Check sheet for the drawn part. Datum: minimum x, y, z corner. Units: mm. A direction names the side the tool comes from. Give positions to 0.01 mm unless a question says otherwise; leave off trailing zeros. Loops run counter-clockwise (first coordinate to the right, second up) from the corner with the lowest first, then second, coordinate; pieces in that order, holes last.
1. Cross-section at C-C, the plane x = 22. Record the cut outline in (y, z).
2. Cross-section at D-D, the plane z = 17. Record the cut outline in (x, y), plus the area to 3 significant figures.
3. Cross-section at A-A, the plane z = 6.5. Record the cut outline in (x, y).
4. Cross-section at B-B, the plane x = 5.5. Record the cut outline in (y, z).
5. Material ranges on L1, parallel to Z at x = 38.5, y = 16.75; L2, parallel to X at y = 11, z = 32; L3, parallel to X at y = 15.75, z = 32, recorded low to high.
6. Go/stop test with flat-tipped pins: pin 1 Ø4.5 at (x, z) = (5.5, 32.5) entering from +Y; pin 2 Ø10.5 at (x, z) = (38, 21) entering from -Y; pin 3 Ø14 at (x, y) = (22, 15) entering from -Z; pin 4 Ø1.5 at (x, z) = (12.5, 8) entering from -Y. Record where each tip stops, or that it passes through.
7. Release check for a two-part mould opening along Y. For the marked faces 4, 5 and 6 record: +Y half, -Y half, draft (parallel to the pull), parting line (faces both ways), or undercut.
8. Tool access check on the marked faces 1, 2 and 3. Record the directions out of +Z, -Z, +X, -X, +Y, -Y that give a thin tool (end or side, any length) a straight path to the whole face; none if there is none.
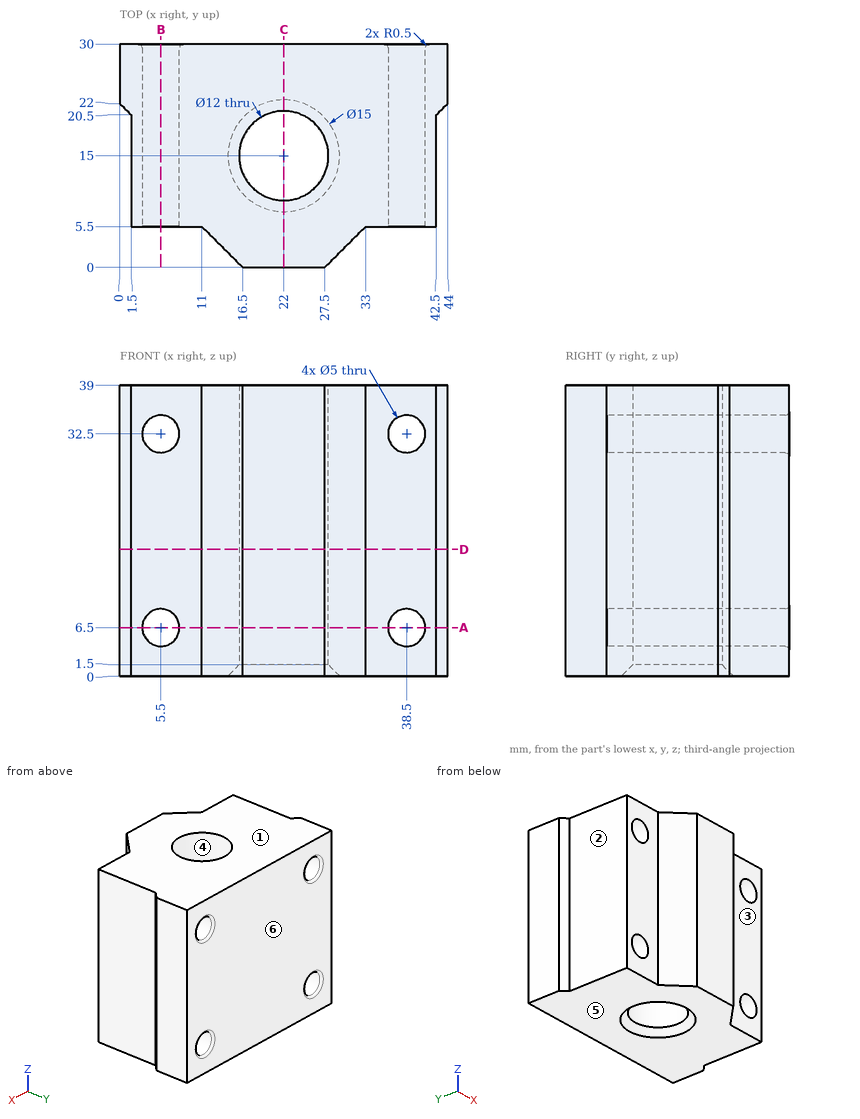
Result:
1. outline: (0, 0) - (7.5, 0) - (9, 1.5) - (9, 39) - (0, 39) - close; (21, 1.5) - (22.5, 0) - (30, 0) - (30, 39) - (21, 39) - close
2. outline: (0, 22) - (1.5, 20.5) - (1.5, 5.5) - (11, 5.5) - (16.5, 0) - (27.5, 0) - (33, 5.5) - (42.5, 5.5) - (42.5, 20.5) - (44, 22) - (44, 30) - (0, 30) - close; hole circle Ø12 at (22, 15)
2. area: 1,010 mm2
3. outline: (0, 22) - (1.5, 20.5) - (1.5, 5.5) - (3, 5.5) - (3, 29.5) arc R0.5 ccw to (2.5, 30) - (0, 30) - close; (8, 5.5) - (11, 5.5) - (16.5, 0) - (27.5, 0) - (33, 5.5) - (36, 5.5) - (36, 29.5) arc R0.5 ccw to (35.5, 30) - (8.5, 30) arc R0.5 ccw to (8, 29.5) - close; (41, 5.5) - (42.5, 5.5) - (42.5, 20.5) - (44, 22) - (44, 30) - (41.5, 30) arc R0.5 ccw to (41, 29.5) - close; hole circle Ø12 at (22, 15)
4. outline: (5.5, 0) - (30, 0) - (30, 3.5) arc R0.5 ccw to (29.5, 4) - (5.5, 4) - close; (5.5, 9) - (29.5, 9) arc R0.5 ccw to (30, 9.5) - (30, 29.5) arc R0.5 ccw to (29.5, 30) - (5.5, 30) - close; (5.5, 35) - (29.5, 35) arc R0.5 ccw to (30, 35.5) - (30, 39) - (5.5, 39) - close
5. L1: z = 0 to 4, 9 to 30, 35 to 39
5. L2: x = 1.5 to 3.05, 7.95 to 17.53, 26.47 to 36.05, 40.95 to 42.5
5. L3: x = 1.5 to 3.05, 7.95 to 16.05, 27.95 to 36.05, 40.95 to 42.5
6. pin 1: passes through
6. pin 2: stops at y = 5.25
6. pin 3: stops at z = 0.5
6. pin 4: stops at y = 3.25
7. face 4: undercut
7. face 5: draft
7. face 6: +Y half
8. face 1: +Z, +X, -X, +Y, -Y
8. face 2: +Z, -Z, -X, -Y
8. face 3: +Z, -Z, +X, -Y
